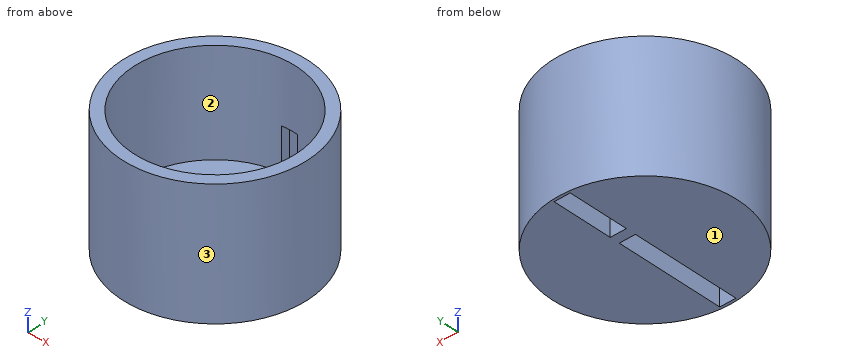
```python
from build123d import *

# Parameters (mm, degrees)
ESQUISSE1_R             = 16
BOSS_EXTRU_1_DEPTH      = 22
ESQUISSE2_W             = 2.8
ESQUISSE2_H             = 31
ENL_V_MAT_EXTRU_1_DEPTH = 11.41
ESQUISSE3_W             = 2.8
ESQUISSE3_H             = 1.7
BOSS_EXTRU_2_DEPTH      = 5
ESQUISSE4_R             = 14
ENL_V_MAT_EXTRU_2_DEPTH = 18


with BuildPart() as part:
    # Esquisse1 → Boss.-Extru.1 (new body)
    with BuildSketch(Plane.XY):
        Circle(ESQUISSE1_R)
    extrude(amount=BOSS_EXTRU_1_DEPTH)

    # Esquisse2 → Enlèv. mat.-Extru.1 (cut)
    with BuildSketch(Plane.XY):
        Rectangle(ESQUISSE2_W, ESQUISSE2_H)
    extrude(amount=ENL_V_MAT_EXTRU_1_DEPTH, mode=Mode.SUBTRACT)

    # Esquisse3 → Boss.-Extru.2 (add)
    with BuildSketch(Plane(origin=(0, 0, 0), x_dir=(-1, 0, 0), z_dir=(0, 0, -1))):
        with Locations((0, 4.15)):
            Rectangle(ESQUISSE3_W, ESQUISSE3_H)
    extrude(amount=-BOSS_EXTRU_2_DEPTH)

    # Esquisse4 → Enlèv. mat.-Extru.2 (cut)
    with BuildSketch(Plane.XY.offset(22)):
        Circle(ESQUISSE4_R)
    extrude(amount=-ENL_V_MAT_EXTRU_2_DEPTH, mode=Mode.SUBTRACT)


solid = part.part
```
Build history of the part. All positions in model axes, mm. Face numbers are marked on the shaded views. Give positions to 0.01 mm unless a question says otherwise; leave off trailing zeros. Loops run counter-clockwise (first coordinate to the right, second up) from the corner with the lowest first, then second, coordinate; pieces in that order, holes last. Notation, with made-up numbers: (48.5, 39) -> (103.5, 39) arc R21 ccw to (103.5, 52) -> close; hole circle Ø8 at (66, 65). An arc over 180 degrees is marked (long way). One line per question, with ' | ' between items.
Q1. Cut at A-A, the plane x = 0. Write the cut outline in (y, z), plus the area to 3 significant figures.
Filled sheet:
outline: (-16, 0) -> (-15.5, 0) -> (-15.5, 11.41) -> (-14, 11.41) -> (-14, 22) -> (-16, 22) -> close; (3.3, 0) -> (5, 0) -> (5, 4) -> (3.3, 4) -> close; (14, 11.41) -> (15.5, 11.41) -> (15.5, 0) -> (16, 0) -> (16, 22) -> (14, 22) -> close | area: 60.6 mm²
Q2. Drill centre lines: line 1 along Y through (x, z) = (0, 8); line 2 along Y through (x, z) = (0, 12.25); line 3 along Z through (x, y) = (-6.5, 8.5). Where is each one in solid material? Low to high. Write a range as [from, to].
Filled sheet:
line 1: y = [-16, -15.5], [15.5, 16] | line 2: y = [-16, -14], [14, 16] | line 3: z = [0, 4]
Q3. Drop flat-ended pins along their axis: pin 1 (3 mm diameter, centred on y = -3.5, z = 6.5, fed in from +X); pin 2 (0.8 mm diameter, centred on x = -0.5, z = 1.5, fed in from -Y); pin 3 (10 mm diameter, centred on y = 10.5, z = 11, fed in from +X) (3 decimals); pin 4 (2 mm diameter, centred on y = -4.5, z = 15.5, fed in from +X). Give the stop position or say it passes through.
Filled sheet:
pin 1: stops at x = 15.87 | pin 2: stops at y = -16 | pin 3: stops at x = 15.025 | pin 4: stops at x = 15.61
Q4. Cut at D-D, the plane x = 12. Write the cut outline in (y, z), plus the area to 3 significant figures.
Filled sheet:
outline: (-10.58, 0) -> (10.58, 0) -> (10.58, 22) -> (7.21, 22) -> (7.21, 4) -> (-7.21, 4) -> (-7.21, 22) -> (-10.58, 22) -> close | area: 206 mm²
Q5. Cut at B-B, the plane z = 5.25. Write the cut outline in (x, y), plus the area to 3 significant figures.
Filled sheet:
outline: circle Ø32 at (0, 0); hole (-1.4, -15.5) -> (1.4, -15.5) -> (1.4, -13.93) arc R14 ccw to (1.4, 13.93) -> (1.4, 15.5) -> (-1.4, 15.5) -> (-1.4, 13.93) arc R14 ccw to (-1.4, -13.93) -> close | area: 180 mm²
Q6. Cut at C-C, the plane y = 0. Write the cut outline in (x, z), plus the area to 3 significant figures.
Filled sheet:
outline: (-16, 0) -> (-1.4, 0) -> (-1.4, 4) -> (-14, 4) -> (-14, 22) -> (-16, 22) -> close; (1.4, 0) -> (16, 0) -> (16, 22) -> (14, 22) -> (14, 4) -> (1.4, 4) -> close | area: 189 mm²
Q7. Pull direction Y, two halves, no side cores. Call the marked faces 1, 2 and 3: pulls with the +Y half, pulls with the -Y half, needs draft (parallel to the pull), parting line crosses it, or undercut.
Filled sheet:
face 1: needs draft | face 2: undercut | face 3: parting line crosses it
